Input: dimensioned drawing with shaded views. Units: mm. Origin: part minimum x, y, z. Coordinates: 2 decimals unless noted, no trailing zeros. Order: outer loops, then holes, each group sorted by start corner. A loop starts at its lowest first (then second) coordinate and runs counter-clockwise, first axis right, second up. Notation, with made-up numbers: M -22,58.25 L -5,58.25 A15 ccw -5,83.25 Z; hole C 51,65.25 d7. An arc over 180 degrees is marked long. Use CSV: the item, a comma, the result in double quotes. Start each with the question number.
1. Material intervals for line 1 (Y direction, x = 117.5, z = 1.35); line 2 (Y direction, x = 181.5, z = 2.45); line 3 (X direction, y = 121, z = 0.35), sorted ascending.
2. Section query A-A on y = 58. Return the cut outline in (x, z).
3. Section query C-C on z = 0.95. Return the cut outline in (x, y), and give its area (3 significant figures).
4. Section query B-B on x = 70.5. Return the cut outline in (y, z).
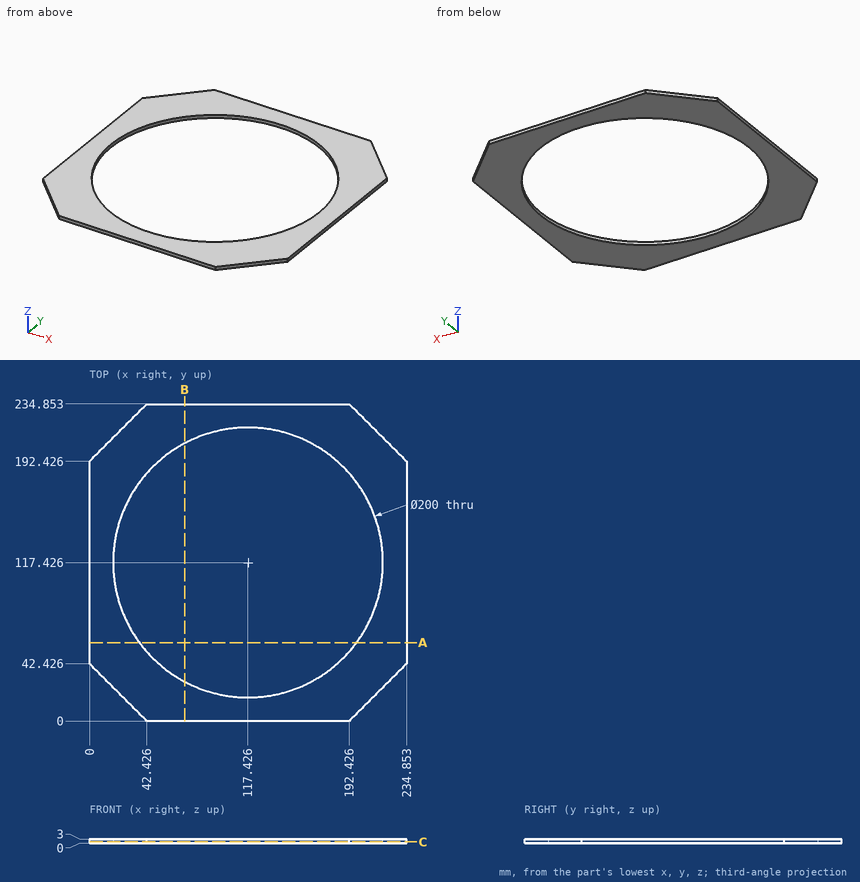
Results list:
1,line 1,"y = 0 to 17.43, 217.43 to 234.85"
1,line 2,"y = 0 to 40.65, 194.2 to 234.85"
1,line 3,"x = 0 to 17.49, 217.36 to 234.85"
2,outline,"M 0,0 L 37,0 L 37,3 L 0,3 Z; M 197.85,0 L 234.85,0 L 234.85,3 L 197.85,3 Z"
3,outline,"M 0,42.43 L 42.43,0 L 192.43,0 L 234.85,42.43 L 234.85,192.43 L 192.43,234.85 L 42.43,234.85 L 0,192.43 Z; hole C 117.43,117.43 d200"
3,area,"20,100 mm²"
4,outline,"M 0,0 L 29.12,0 L 29.12,3 L 0,3 Z; M 205.73,0 L 234.85,0 L 234.85,3 L 205.73,3 Z"
